Model file for the job. Use its own axes, mm. Coordinates: 2 decimals unless noted, no trailing zeros. Write each loop counter-clockwise with the first axis right and the second up, starting at its lowest first coordinate (ties: lowest second). Pieces come first, ordered by that corner, then holes. Notation, with made-up numbers: M -35,-30 L -4,-30 A22 cw -4,-20 Z; hole C 24,59.5 d10. An arc over 180 degrees is marked long. Answer in a Markdown table with one row per item. Add a question column.
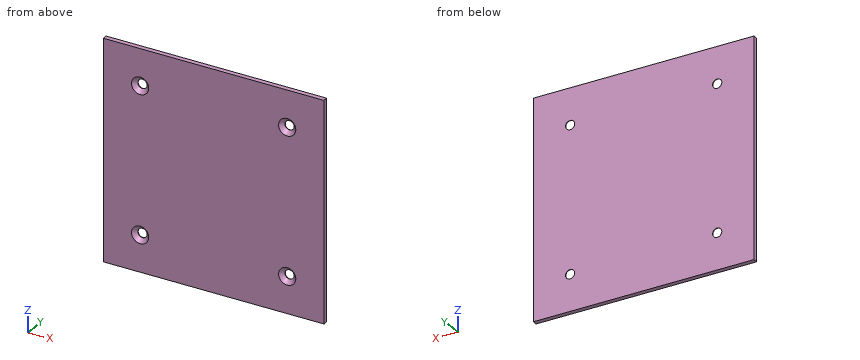
```python
from build123d import *

# Parameters (mm, degrees)
F0_W           = 304.8
F0_H           = 304.8
F1_DEPTH       = 6.35
F3_D           = 12.7
F3_CSINK_D     = 23.8252
F3_CSINK_ANGLE = 90


with BuildPart() as f1:
    # F0 (on Front) → F1 (new body)
    with BuildSketch(Plane.XZ):
        Rectangle(F0_W, F0_H)
    extrude(amount=F1_DEPTH)

    # F3 (through all)
    with Locations(Plane.XZ.offset(6.35)):
        with Locations((-101.6, 101.6), (101.6, 101.6), (101.6, -101.6), (-101.6, -101.6)):
            CounterSinkHole(F3_D / 2, F3_CSINK_D / 2, counter_sink_angle=F3_CSINK_ANGLE)


solid = f1.part
```
1) Slice it at B-B (z = 101.6). Give the cut face in (x, y).
2) Slice it at A-A (x = -101.6). Give the cut face in (y, z).
3) Flat gauge pins, fed straight in: pin 1 Ø12 at (x, z) = (62.5, -32.5) entering from +Y; pin 2 Ø10 at (x, z) = (101.6, 101.6) entering from -Y (1 decimal). Where does each tip first touch, or does it go through?
4) Drill centre line: probe 1 along X at (y, z) = (-0.2, -101.6). Where is it in solid material? Low to high.
Ans:
| question | item | result |
|---|---|---|
| 1 | outline | M -152.4,-6.35 L -113.51,-6.35 L -107.95,-0.79 L -107.95,0 L -152.4,0 Z; M -95.25,-0.79 L -89.69,-6.35 L 89.69,-6.35 L 95.25,-0.79 L 95.25,0 L -95.25,0 Z; M 107.95,-0.79 L 113.51,-6.35 L 152.4,-6.35 L 152.4,0 L 107.95,0 Z |
| 2 | outline | M -6.35,-152.4 L 0,-152.4 L 0,-107.95 L -0.79,-107.95 L -6.35,-113.51 Z; M -6.35,-89.69 L -0.79,-95.25 L 0,-95.25 L 0,95.25 L -0.79,95.25 L -6.35,89.69 Z; M -6.35,113.51 L -0.79,107.95 L 0,107.95 L 0,152.4 L -6.35,152.4 Z |
| 3 | pin 1 | stops at y = 0 |
| 3 | pin 2 | passes through |
| 4 | probe 1 | x = -152.4 to -107.95, -95.25 to 95.25, 107.95 to 152.4 |
